Study the drawing (mm; zero at the part's minimum x, y, z) and answer. A direction names the side the tool comes from. Coordinates: 2 decimals unless noted, no trailing zeros. Loops run counter-clockwise (first coordinate to the right, second up) from the corner with the lowest first, then second, coordinate; pieces in that order, holes last. Notation, with made-up numbers: (3, 5.25) - (23, 5.25) arc R37 ccw to (23, 44.25) - close; hole circle Ø3 at (0, 10). An arc over 180 degrees is marked (long way). Use CSV: the item, a comma, the result in double quotes.
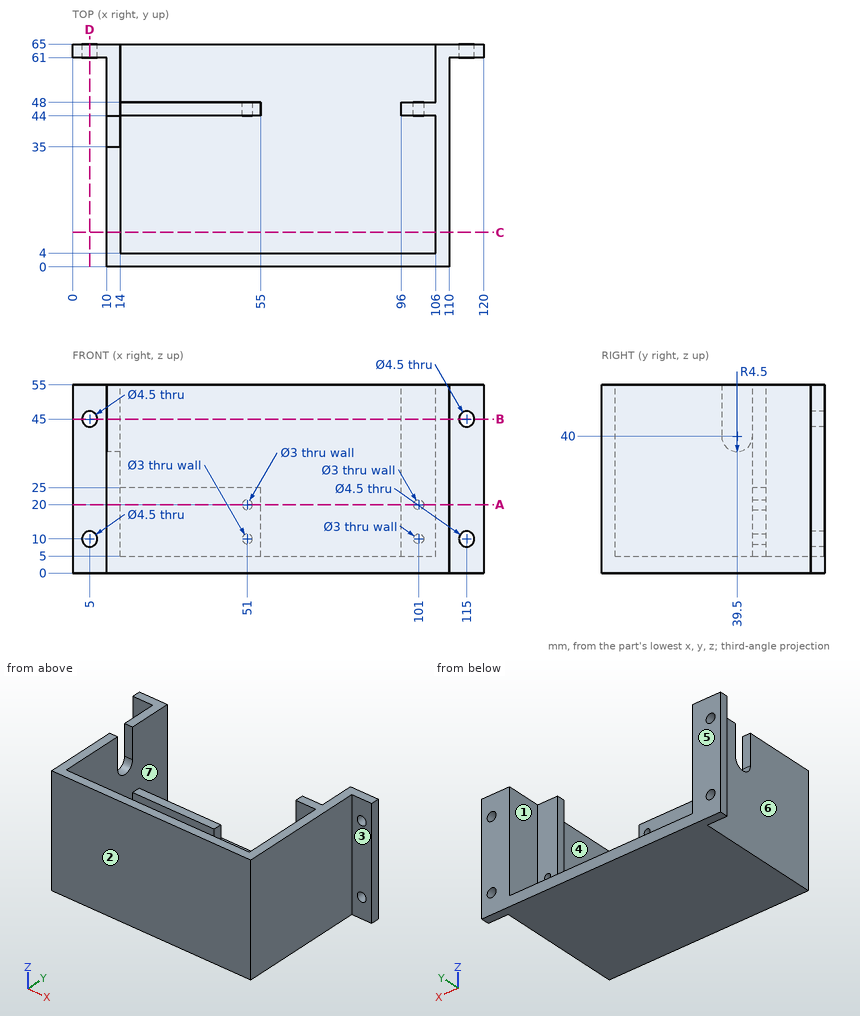
Q1. The part is cut by section A-A on z = 20. Determine the outline of the cut face in (x, y), and give its area (3 significant figures).
Reported:
outline,"(0, 61) - (10, 61) - (10, 0) - (110, 0) - (110, 61) - (120, 61) - (120, 65) - (106, 65) - (106, 48) - (102.5, 48) - (102.5, 44) - (106, 44) - (106, 4) - (14, 4) - (14, 44) - (49.5, 44) - (49.5, 48) - (14, 48) - (14, 65) - (0, 65) - close; (52.5, 44) - (55, 44) - (55, 48) - (52.5, 48) - close; (96, 44) - (99.5, 44) - (99.5, 48) - (96, 48) - close"
area,"1,150 mm²"
Q2. The part is cut by section D-D on x = 5. Determine the outline of the cut face in (y, z).
Reported:
outline,"(61, 0) - (65, 0) - (65, 7.75) - (61, 7.75) - close; (61, 12.25) - (65, 12.25) - (65, 42.75) - (61, 42.75) - close; (61, 47.25) - (65, 47.25) - (65, 55) - (61, 55) - close"
Q3. For a pull along X with two mould halves and no side action, classify the marked faces 4, 5, 6 and 7 as +X half, -X half, draft (parallel to the pull), parting line (faces both ways), or undercut.
Reported:
face 4,"undercut"
face 5,"draft"
face 6,"-X half"
face 7,"undercut"
Q4. Given P1, Ø5, axis at y = 13.5, z = 7, coming from the +X side; P2, Ø4, axis at x = 101, z = 10, coming from the +Y side; P3, Ø5, axis at y = 55.5, z = 36.5, coming from the -X side, each flat-ended and moving along its own axis, determine where each tip first touches the part or whether it passes through.
Reported:
P1,"stops at x = 110"
P2,"stops at y = 48"
P3,"stops at x = 10"
Q5. The part is cut by section B-B on z = 45. Determine the outline of the cut face in (x, y), and give its area (3 significant figures).
Reported:
outline,"(0, 61) - (2.75, 61) - (2.75, 65) - (0, 65) - close; (7.25, 61) - (10, 61) - (10, 44) - (14, 44) - (14, 65) - (7.25, 65) - close; (10, 0) - (110, 0) - (110, 61) - (112.75, 61) - (112.75, 65) - (106, 65) - (106, 48) - (96, 48) - (96, 44) - (106, 44) - (106, 4) - (14, 4) - (14, 35) - (10, 35) - close; (117.25, 61) - (120, 61) - (120, 65) - (117.25, 65) - close"
area,"936 mm²"
Q6. The part is cut by section C-C on y = 10. Determine the outline of the cut face in (x, z), and give its area (3 significant figures).
Reported:
outline,"(10, 0) - (110, 0) - (110, 55) - (106, 55) - (106, 5) - (14, 5) - (14, 55) - (10, 55) - close"
area,"900 mm²"
Q7. Find the intervals of material crossed by probe 1 along X at (y, z) = (45.15, 10); probe 2 along Z at (x, y) = (101, 45.55); probe 3 along X at (y, z) = (24, 12.5), in increasing order. Write a range as [from, to].
Reported:
probe 1,"x = [10, 49.5], [52.5, 55], [96, 99.5], [102.5, 110]"
probe 2,"z = [0, 8.5], [11.5, 18.5], [21.5, 55]"
probe 3,"x = [10, 14], [106, 110]"
Q8. A tool of negligible diameter and unlimited length cuts with its end or side. For the marked faces 1, 2 and 3, from which of +Z, -Z, +X, -X, +Y, -Y can it reach the whole face along a straight path? Write none if from no direction.
Reported:
face 1,"+Z, +Y"
face 2,"+Z, -Z, +X, -X, -Y"
face 3,"+Z, -Z, +X, -Y"
